Job drawing, mm, ordinate dimensions from the low corner. One solid piece. Give positions to 0.01 mm unless a question says otherwise; leave off trailing zeros. Write each loop counter-clockwise with the first axis right and the second up, starting at its lowest first coordinate (ties: lowest second). Pieces come first, ordered by that corner, then holes. Notation, with made-up numbers: M 6.5,-35.75 L 57.5,-35.75 A8 ccw 57.5,-25.75 Z; hole C -22.75,36 d6. An arc over 180 degrees is marked long. Use CSV: the item, a comma, the result in double quotes. Start each with the question number.
Item 1: Cut at D-D (y = 14.45). List the corners of the cut face in (x, z), then the cut area to 4 significant figures.
Item 2: Drill centre lines: line 1 (X direction, y = 45, z = 17); line 2 (X direction, y = 16, z = 4); line 3 (X direction, y = 46.5, z = 9). Where is each one in solid material? Low to high. Write a range as [from, to].
Item 3: Cut at A-A (y = 45.45). List the corners of the cut face in (x, z).
Item 4: Cut at B-B (x = 169). List the corners of the cut face in (y, z), then the cut area to 3 significant figures.
Item 5: Pin check, flat tips, straight feed: pin 1 (7 mm diameter, centred on x = 15, y = 14.45, fed in from +Z); pin 2 (4 mm diameter, centred on x = 30.5, z = 17, fed in from -Y); pin 3 (6 mm diameter, centred on x = 9.56, z = 9, fed in from +Y). Stop position of each tip, or through.
Item 6: Cut at C-C (z = 27). List the corners of the cut face in (x, y), then the cut area to 3 significant figures.
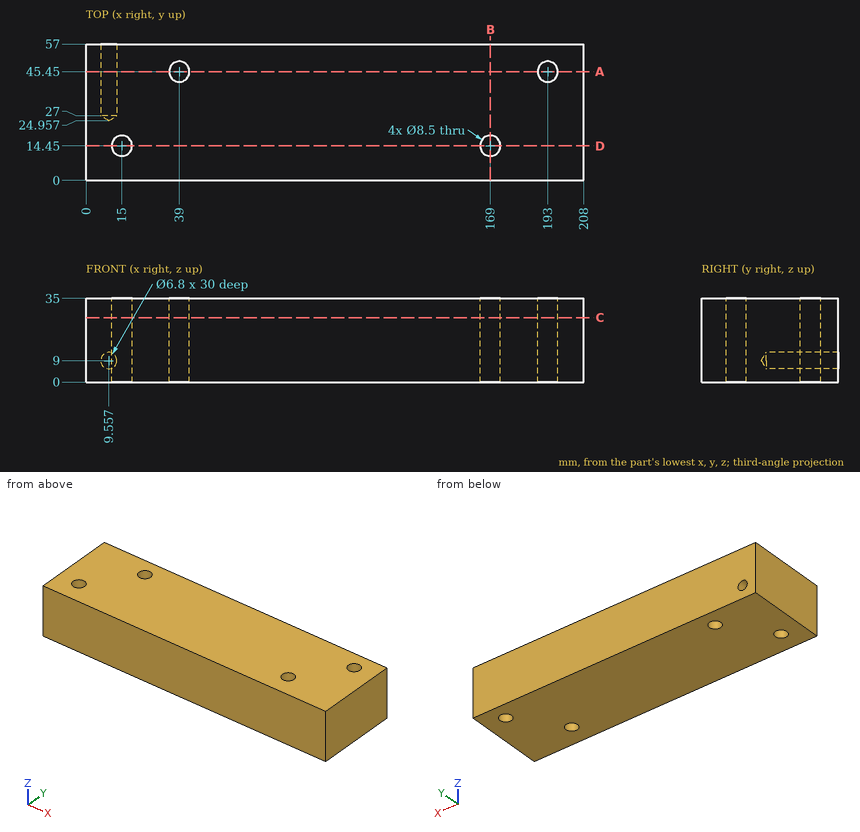
Worked answers:
1,outline,"M 0,0 L 10.75,0 L 10.75,35 L 0,35 Z; M 19.25,0 L 164.75,0 L 164.75,35 L 19.25,35 Z; M 173.25,0 L 208,0 L 208,35 L 173.25,35 Z"
1,area,"6,685 mm^2"
2,line 1,"x = [0, 34.77], [43.23, 188.77], [197.23, 208]"
2,line 2,"x = [0, 11.04], [18.96, 165.04], [172.96, 208]"
2,line 3,"x = [0, 6.16], [12.96, 34.88], [43.12, 188.88], [197.12, 208]"
3,outline,"M 0,0 L 34.75,0 L 34.75,35 L 0,35 Z; M 43.25,0 L 188.75,0 L 188.75,35 L 43.25,35 Z; M 197.25,0 L 208,0 L 208,35 L 197.25,35 Z; hole C 9.56,9 d6.8"
4,outline,"M 0,0 L 10.2,0 L 10.2,35 L 0,35 Z; M 18.7,0 L 57,0 L 57,35 L 18.7,35 Z"
4,area,"1,700 mm^2"
5,pin 1,"passes through"
5,pin 2,"stops at y = 0"
5,pin 3,"stops at y = 26.76"
6,outline,"M 0,0 L 208,0 L 208,57 L 0,57 Z; hole C 15,14.45 d8.5; hole C 39,45.45 d8.5; hole C 169,14.45 d8.5; hole C 193,45.45 d8.5"
6,area,"11,600 mm^2"
